CAD build for the part. Positions are in the model's coordinates, mm. A direction names the side the tool comes from. Round coordinates to 2 decimals unless told otherwise and drop trailing zeros. Write each loop counter-clockwise with the first axis right and the second up, starting at its lowest first coordinate (ties: lowest second). Pieces come first, ordered by that corner, then holes. Notation, with made-up numbers: M 89.25,63 L 108.25,63 A24 cw 108.25,78 Z; hole C 74.25,2.25 d8. An arc over 180 degrees is marked long. Write each question's results on one line, items separated by ' | '. Start each with the question number.
```python
from build123d import *

# Parameters (mm, degrees)
SKIZZE1_W                       = 65
SKIZZE1_H                       = 50
AUFSATZ_LINEAR_AUSTRAGEN1_DEPTH = 3
SKIZZE2_W                       = 58
SKIZZE2_H                       = 43
AUFSATZ_LINEAR_AUSTRAGEN2_DEPTH = 3
SKIZZE7_W                       = 35.2
SKIZZE7_H                       = 4.5
SCHNITT_LINEAR_AUSTRAGEN2_DEPTH = 58
SKIZZE9_W                       = 1
SKIZZE9_H                       = 31.2
SCHNITT_LINEAR_AUSTRAGEN3_DEPTH = 52
SCHNITT_LINEAR_AUSTRAGEN4_REACH = 8
SKIZZE10_W                      = 38.3
SKIZZE10_H                      = 32.1
VERRUNDUNG2_R                   = 3
SKIZZE11_R                      = 1
SCHNITT_LINEAR_AUSTRAGEN5_DEPTH = 7
FASE1_SIZE                      = 0.5


with BuildPart() as part:
    # Skizze1 → Aufsatz-Linear austragen1 (new body)
    with BuildSketch(Plane.XY):
        with Locations((32.5, -25)):
            Rectangle(SKIZZE1_W, SKIZZE1_H)
    extrude(amount=AUFSATZ_LINEAR_AUSTRAGEN1_DEPTH)

    # Skizze2 → Aufsatz-Linear austragen2 (add)
    with BuildSketch(Plane.XY.offset(3)):
        with Locations((32.5, -25)):
            Rectangle(SKIZZE2_W, SKIZZE2_H)
    extrude(amount=AUFSATZ_LINEAR_AUSTRAGEN2_DEPTH)

    # Skizze7 → Schnitt-Linear austragen2 (cut)
    with BuildSketch(Plane(origin=(65, -65, 0), x_dir=(0, 1, 0), z_dir=(-1, 0, 0))):
        with Locations((40, -2.75)):
            Rectangle(SKIZZE7_W, SKIZZE7_H)
    extrude(amount=SCHNITT_LINEAR_AUSTRAGEN2_DEPTH, mode=Mode.SUBTRACT)

    # Skizze9 → Schnitt-Linear austragen3 (cut)
    with BuildSketch(Plane(origin=(61.5, 0, 0), x_dir=(0, 0, -1), z_dir=(1, 0, 0))):
        with Locations((-5.5, -25)):
            Rectangle(SKIZZE9_W, SKIZZE9_H)
    extrude(amount=-SCHNITT_LINEAR_AUSTRAGEN3_DEPTH, mode=Mode.SUBTRACT)

    # Skizze10 → Schnitt-Linear austragen4 (cut, up to next)
    with BuildSketch(Plane(origin=(0, 0, 0), x_dir=(-1, 0, 0), z_dir=(0, 0, -1)), mode=Mode.PRIVATE) as schnitt_linear_austragen4_sk1:
        with Locations((-32.5, -25)):
            Rectangle(SKIZZE10_W, SKIZZE10_H)
    schnitt_linear_austragen4_tool1 = extrude(schnitt_linear_austragen4_sk1.sketch, amount=-SCHNITT_LINEAR_AUSTRAGEN4_REACH, mode=Mode.PRIVATE) & part.part
    add(schnitt_linear_austragen4_tool1.solids().sort_by_distance((32.5, -25, 0))[0], mode=Mode.SUBTRACT)

    # Verrundung2
    verrundung2_edges = [part.edges().sort_by_distance(p)[0] for p in [
        (61.5, -3.5, 4.5),
        (3.5, -3.5, 4.5),
        (3.5, -46.5, 4.5),
        (61.5, -46.5, 4.5),
        (0, 0, 1.5),
        (65, 0, 1.5),
        (65, -50, 1.5),
        (0, -50, 1.5),
    ]]
    fillet(verrundung2_edges, radius=VERRUNDUNG2_R)

    # Skizze11 → Schnitt-Linear austragen5 (cut, through all)
    with BuildSketch(Plane(origin=(0, 0, 0), x_dir=(-1, 0, 0), z_dir=(0, 0, -1))):
        with Locations((-63, -2)):
            Circle(SKIZZE11_R)
        with Locations((-2, -2)):
            Circle(SKIZZE11_R)
        with Locations((-2, -48)):
            Circle(SKIZZE11_R)
        with Locations((-63, -48)):
            Circle(SKIZZE11_R)
    extrude(amount=-SCHNITT_LINEAR_AUSTRAGEN5_DEPTH, mode=Mode.SUBTRACT)

    # Fase1
    fase1_edges = [part.edges().sort_by_distance(p)[0] for p in [
        (64, -2, 0),
        (3, -2, 0),
        (3, -48, 0),
        (64, -48, 0),
    ]]
    chamfer(fase1_edges, length=FASE1_SIZE)


solid = part.part
```
1) Pull direction Y, two halves, no side cores. Call faces 1 (the face through (7, -25, 3)), 2 (the face through (61.5, -43, 5)), 3 (the face through (64.1, -49.14, 1.52)), 4 (the face through (32, 0, 1)): pulls with the +Y half, pulls with the -Y half, needs draft (parallel to the pull), parting line crosses it, or undercut.
2) Saw through at B-B, the plane z = 1.55. Write the cut outline in (x, y), plus the area to 3 significant figures.
3) 3-axis set-ups, long thin cutter, end or side, ignore diameter. For faces 5 (the face through (60.64, -4.4, 4.52)), 6 (the face through (3.5, -25, 4)), 7 (the face through (36, -42.6, 3)): which of +Z, -Z, +X, -X, +Y, -Y reach the whole face in a straight line?
4) Saw through at C-C, the plane x = 63. Write the cut outline in (y, z), plus the area to 3 significant figures.
5) Wall check: line 1 along Y through (x, z) = (2, 1.7); line 2 along Z through (x, y) = (9, -25); line 3 along Y through (x, z) = (63, 1.55). Give the ranges that are in metal, low to high. Write a range as from..to.
6) Saw through at A-A, the plane y = -30. Write the cut outline in (x, z).
7) Drop flat-ended pins along their axis: pin 1 Ø1.1 at (y, z) = (-19, 5.5) entering from +X; pin 2 Ø1.5 at (y, z) = (-8, 5) entering from +X; pin 3 Ø1.8 at (x, y) = (2, -48) entering from -Z; pin 4 Ø3 at (x, z) = (8, 5.5) entering from +Y. Give the stop position or say it passes through.
8) Saw through at D-D, the plane y = -2. Write the cut outline in (x, z).
Filled sheet:
1) face 1: undercut | face 2: needs draft | face 3: pulls with the -Y half | face 4: pulls with the +Y half
2) outline: M 0,-47 A3 ccw 3,-50 L 62,-50 A3 ccw 65,-47 L 65,-42.6 L 7,-42.6 L 7,-7.4 L 65,-7.4 L 65,-3 A3 ccw 62,0 L 3,0 A3 ccw 0,-3 Z; hole C 2,-48 d2; hole C 2,-2 d2; hole C 63,-48 d2; hole C 63,-2 d2 | area: 1,190 mm^2
3) face 5: +Z, +X, +Y | face 6: +Z, -X, +Y, -Y | face 7: +X
4) outline: M -49.83,0 L -49.5,0 L -49,0.5 L -49,3 L -49.83,3 Z; M -47,0.5 L -46.5,0 L -3.5,0 L -3,0.5 L -3,3 L -7.4,3 L -7.4,0.5 L -42.6,0.5 L -42.6,3 L -47,3 Z; M -1,0.5 L -0.5,0 L -0.17,0 L -0.17,3 L -1,3 Z | area: 48.5 mm^2
5) line 1: y = -49.83..-49, -47..-3, -1..-0.17 | line 2: z = 0..0.5, 5..6 | line 3: y = -49.83..-49, -47..-42.6, -7.4..-3, -1..-0.17
6) outline: M 0,0 L 13.35,0 L 13.35,0.5 L 7,0.5 L 7,5 L 9.5,5 L 9.5,6 L 3.5,6 L 3.5,3 L 0,3 Z; M 51.65,0 L 65,0 L 65,0.5 L 51.65,0.5 Z
7) pin 1: stops at x = 9.5 | pin 2: stops at x = 61.5 | pin 3: passes through | pin 4: stops at y = -3.5
8) outline: M 0.17,0 L 0.5,0 L 1,0.5 L 1,3 L 0.17,3 Z; M 3,0.5 L 3.5,0 L 61.5,0 L 62,0.5 L 62,3 L 3,3 Z; M 64,0.5 L 64.5,0 L 64.83,0 L 64.83,3 L 64,3 Z
